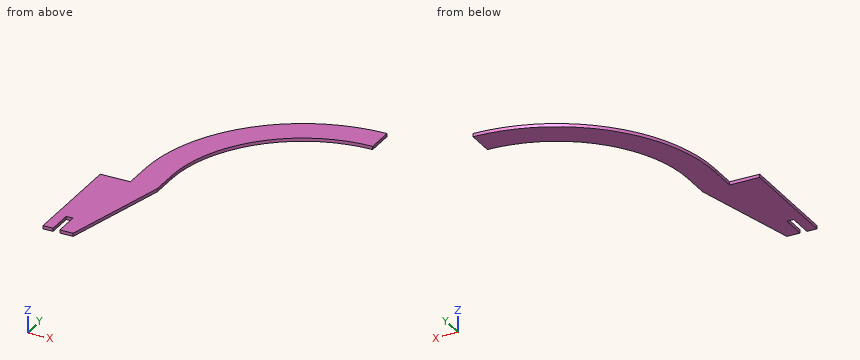
```python
from build123d import *

# Parameters (mm, degrees)
BOSS_EXTRUDE1_DEPTH = 18.25625


with BuildPart() as part:
    # Sketch1 → Boss-Extrude1 (new body)
    with BuildSketch(Plane.XY):
        with BuildLine():
            Line((-1416.065070695, 421.537507263), (-1416.065070695, -188.062492737))
            Line((-1416.065070695, -188.062492737), (-1358.915070695, -188.062492737))
            Line((-1358.915070695, -188.062492737), (-1358.915070695, -48.362492737))
            Line((-1358.915070695, -48.362492737), (-1320.815070695, -48.362492737))
            Line((-1320.815070695, -48.362492737), (-1320.815070695, -188.062492737))
            Line((-1320.815070695, -188.062492737), (-1245.720896666, -188.062492737))
            Line((-1245.720896666, -188.062492737), (-1093.320896666, 421.537507263))
            Line((-1093.320896666, 421.537507263), (-1093.320896666, 573.937507263))
            ThreePointArc((-1093.320896666, 573.937507263), (-875.715879749, 1099.282490346), (-350.370896666, 1316.887507263))
            Line((-350.370896666, 1316.887507263), (-350.370896666, 1469.287507263))
            ThreePointArc((-350.370896666, 1469.287507263), (-983.478953202, 1207.045563799), (-1245.720896666, 573.937507263))
            Line((-1245.720896666, 573.937507263), (-1245.720896666, 421.537507263))
            Line((-1245.720896666, 421.537507263), (-1416.065070695, 421.537507263))
        make_face()
    extrude(amount=BOSS_EXTRUDE1_DEPTH)


solid = part.part
```
Check sheet for the modelled part. Datum: model origin and axes. Units: mm. Round coordinates to 2 decimals unless told otherwise and drop trailing zeros. Loops run counter-clockwise (first coordinate to the right, second up) from the corner with the lowest first, then second, coordinate; pieces in that order, holes last. Notation, with made-up numbers: (30, -10) -> (63, -10) arc R18 ccw to (63, 0) -> close; hole circle Ø7 at (84.25, 4). An arc over 180 degrees is marked (long way). Write item = value, one per line. Start each with the question number.
1) Thickness scan on probe 1 along Y at (x, z) = (-1316, 5.25); probe 2 along X at (y, z) = (581, 9.75); probe 3 along X at (y, z) = (576.5, 8.25). Record the ranges inside material, lowest first.
2) Gauge pin test, flat ends, axial feed: pin 1 Ø5.5 at (y, z) = (-92.5, 10.5) entering from +X; pin 2 Ø5 at (y, z) = (790, 10.5) entering from -X; pin 3 Ø2 at (x, z) = (-896, 14.5) entering from +Y. Record the tip position at first contact, or that the pin passes through.
3) Sectioned sample at A-A, the plane z = 13.5. Record the cut outline in (x, y).
4) Sectioned sample at B-B, the plane y = 508.5. Record the cut outline in (x, z).
5) Sectioned sample at C-C, the plane x = -1069.5. Record the cut outline in (y, z), plus the area to 3 significant figures.
Results are:
q1.probe_1 = -188.06 to 421.54
q1.probe_2 = -1245.69 to -1093.29
q1.probe_3 = -1245.72 to -1093.32
q2.pin_1 = -1221.14
q2.pin_2 = -1219.88
q2.pin_3 = 1284.59
q3.outline = (-1416.07, -188.06) -> (-1358.92, -188.06) -> (-1358.92, -48.36) -> (-1320.82, -48.36) -> (-1320.82, -188.06) -> (-1245.72, -188.06) -> (-1093.32, 421.54) -> (-1093.32, 573.94) arc R742.95 cw to (-350.37, 1316.89) -> (-350.37, 1469.29) arc R895.35 ccw to (-1245.72, 573.94) -> (-1245.72, 421.54) -> (-1416.07, 421.54) -> close
q4.outline = (-1245.72, 0) -> (-1093.32, 0) -> (-1093.32, 18.26) -> (-1245.72, 18.26) -> close
q5.outline = (760.56, 0) -> (1107.33, 0) -> (1107.33, 18.26) -> (760.56, 18.26) -> close
q5.area = 6,330 mm^2
